```python
from build123d import *

# Parameters (mm, degrees)
BOSS_EXTRUDE1_DEPTH = 10
SKETCH2_R           = 3.5
BOSS_EXTRUDE2_DEPTH = 7.5
SKETCH3_W           = 3.16759605
SKETCH3_H           = 3.16756905
CUT_EXTRUDE1_DEPTH  = 5


with BuildPart() as part:
    # Sketch1 → Boss-Extrude1 (new body)
    with BuildSketch(Plane.XY):
        with BuildLine():
            ThreePointArc((-2.449489743, 2.5), (0, -3.5), (2.449489743, 2.5))
            ThreePointArc((2.449489743, 2.5), (0, 3.5), (-2.449489743, 2.5))
        make_face()
        with BuildLine():
            Line((-2, 1.5), (2, 1.5))
            ThreePointArc((2, 1.5), (0, -2.5), (-2, 1.5))
        make_face(mode=Mode.SUBTRACT)
    extrude(amount=BOSS_EXTRUDE1_DEPTH)

    # Sketch2 → Boss-Extrude2 (add)
    with BuildSketch(Plane.XY.offset(10)):
        Circle(SKETCH2_R)
    extrude(amount=BOSS_EXTRUDE2_DEPTH)

    # Sketch3 → Cut-Extrude1 (cut)
    with BuildSketch(Plane.XY.offset(17.5)):
        Rectangle(SKETCH3_W, SKETCH3_H)
    extrude(amount=-CUT_EXTRUDE1_DEPTH, mode=Mode.SUBTRACT)


solid = part.part
```
CAD build for the part. Positions are in the model's coordinates, mm. A direction names the side the tool comes from. Round coordinates to 2 decimals unless told otherwise and drop trailing zeros. Order: outer loops, then holes, each group sorted by start corner. A loop starts at its lowest first (then second) coordinate and runs counter-clockwise, first axis right, second up. Notation, with made-up numbers: (15, 50) - (72, 50) arc R18 cw to (72, 58) - close; hole circle Ø3 at (-11.75, 9). An arc over 180 degrees is marked (long way). Answer in a Markdown table with one row per item. Add a question column.
(1) Band-saw the part on C-C on y = 0. List the corners of the cut face in (x, z).
(2) 3-axis set-ups, long thin cutter, end or side, ignore diameter. For faces 3 (the face through (-2, 0, 17.5)), 4 (the face through (1.584, 0, 15)), 5 (the face through (0, 0, 10)): which of +Z, -Z, +X, -X, +Y, -Y reach the whole face in a straight line?
(3) Drop flat-ended pins along their axis: pin 1 Ø3 at (x, z) = (-2, 6) entering from +Y; pin 2 Ø2 at (y, z) = (2.5, 7) entering from +X. Give the stop position or say it passes through.
(4) Band-saw the part on A-A on x = 0. List the corners of the cut face in (y, z).
(5) Band-saw the part on B-B on z = 4.25. List the corners of the cut face in (x, y).
(6) Probe L1, parallel to X at y = 0, z = 2.5; L2, parallel to Z at x = 1, y = -1.5; L3, parallel to X at y = -2, z = 5. List the from-to ranges inside material, lowest first. Write a range as [from, to].
(7) Band-saw the part on D-D on z = 12.25. List the corners of the cut face in (x, y).
(8) Mould opens along Y. For faces 1 (the face through (0, 0, 12.5)), 2 (the face through (0, 2, 0)) say: +Y half, -Y half, draft (parallel to the pull), parting line (faces both ways), or undercut.
Data:
| question | item | result |
|---|---|---|
| 1 | outline | (-3.5, 0) - (-2.5, 0) - (-2.5, 10) - (2.5, 10) - (2.5, 0) - (3.5, 0) - (3.5, 17.5) - (1.58, 17.5) - (1.58, 12.5) - (-1.58, 12.5) - (-1.58, 17.5) - (-3.5, 17.5) - close |
| 2 | face 3 | +Z, +X, -X, +Y, -Y |
| 2 | face 4 | +Z |
| 2 | face 5 | -Z |
| 3 | pin 1 | stops at y = 3.46 |
| 3 | pin 2 | stops at x = 3.16 |
| 4 | outline | (-3.5, 0) - (-2.5, 0) - (-2.5, 10) - (1.5, 10) - (1.5, 0) - (3.5, 0) - (3.5, 17.5) - (1.58, 17.5) - (1.58, 12.5) - (-1.58, 12.5) - (-1.58, 17.5) - (-3.5, 17.5) - close |
| 5 | outline | circle Ø7 at (0, 0); hole (-2, 1.5) arc R2.5 ccw (long way) to (2, 1.5) - close |
| 6 | L1 | x = [-3.5, -2.5], [2.5, 3.5] |
| 6 | L2 | z = [10, 12.5] |
| 6 | L3 | x = [-2.87, -1.5], [1.5, 2.87] |
| 7 | outline | circle Ø7 at (0, 0) |
| 8 | face 1 | undercut |
| 8 | face 2 | draft |
